Check sheet for the modelled part. Datum: model origin and axes. Units: mm. A direction names the side the tool comes from. Give positions to 0.01 mm unless a question says otherwise; leave off trailing zeros. Write each loop counter-clockwise with the first axis right and the second up, starting at its lowest first coordinate (ties: lowest second). Pieces come first, ordered by that corner, then holes. Notation, with made-up numbers: (-28, 27) -> (18, 27) arc R9 ccw to (18, 38) -> close; hole circle Ø11 at (-29, -31.5). An arc over 180 degrees is marked (long way). Answer as a JSON object with one key per item and string values.
from build123d import *

# Parameters (mm, degrees)
BOSS_EXTRUDE2_DEPTH = 3


with BuildPart() as part:
    # Sketch1 → Boss-Extrude2 (new body)
    with BuildSketch(Plane(origin=(0, 0, 0), x_dir=(1, 0, 0), z_dir=(0, 1, 0))):
        with BuildLine():
            Line((0, 0), (-3.8, 0))
            ThreePointArc((-3.8, 0), (-5.3, 1.5), (-3.8, 3))
            Line((-3.8, 3), (15.47, 3))
            Line((15.47, 3), (15.47, 4.149016738))
            ThreePointArc((15.47, 4.149016738), (14.185724127, 7.49466977), (10.992642316, 9.121626215))
            Line((10.992642316, 9.121626215), (5.783295319, 9.669150648))
            ThreePointArc((5.783295319, 9.669150648), (4.874143319, 10), (4.226657422, 10.718874584))
            ThreePointArc((4.226657422, 10.718874584), (-1.078837134, 13.36), (-5.3, 9.2))
            Line((-5.3, 9.2), (-8.03, 9.2))
            ThreePointArc((-8.03, 9.2), (-15.73, 1.5), (-8.03, -6.2))
            Line((-8.03, -6.2), (-1.5, -6.2))
            ThreePointArc((-1.5, -6.2), (-0.439339828, -5.760660172), (0, -4.7))
            Line((0, -4.7), (0, 0))
        make_face()
    extrude(amount=BOSS_EXTRUDE2_DEPTH)


solid = part.part
1. Sectioned sample at B-B, the plane z = -1.5. Enter the section's corners in (x, y), plus the area to 3 significant figures.
Determined:
{"outline": "(-15.73, 0) -> (-5.3, 0) -> (-5.3, 3) -> (-15.73, 3) -> close", "area": "31.3 mm^2"}
2. Scan lines: L1, parallel to Z at x = -2.5, y = 2.1; L2, parallel to Z at x = 5, y = 2.2; L3, parallel to X at y = 1.15, z = -3.25. Record each from-to range of solid material in increasing order. Write a range as [from, to].
Determined:
{"L1": "[-12.91, -3], [0, 6.2]", "L2": "[-9.92, -3]", "L3": "[-15.53, 15.47]"}
3. Access from +Z, -Z, +X, -X, +Y, -Y to the whole of each face (thin tool, end or side, straight path). Record for faces 1 (the face through (6, 1, -3)), 2 (the face through (-4, 3, -4)), 3 (the face through (4.89, 1.48, -9.99)), 4 (the face through (0, 1, 2)), 5 (the face through (-7, 1, -9.2)).
Determined:
{"face 1": "+X, +Y, -Y", "face 2": "+Z, -Z, +X, -X, +Y", "face 3": "-Z, +X, +Y, -Y", "face 4": "+Z, +X, +Y, -Y", "face 5": "-Z, -X, +Y, -Y"}
4. Mould release check, pull along Z, two halves, no side actions. Record for faces 6 (the face through (-5.3, 1.5, -1.5)), 7 (the face through (-15.73, 1.48, -1.67)), 8 (the face through (-0.45, 1.48, 5.77)), 9 (the face through (-2, 1, 0)): released by +Z, released by -Z, zero draft, split by the parting line, or undercut.
Determined:
{"face 6": "undercut", "face 7": "split by the parting line", "face 8": "released by +Z", "face 9": "undercut"}
5. Go/stop test with flat-tipped pins: P1, Ø1.4, axis at x = -6.5, y = 1, coming from the -Z side; P2, Ø1.5, axis at x = -2.5, y = 2, coming from the -Z side. Record where each tip stops, or that it passes through.
Determined:
{"P1": "z = -9.2", "P2": "z = -13.21"}
6. Sectioned sample at A-A, the plane y = 0.3. Enter the section's corners in (x, z), plus the area to 3 significant figures.
Determined:
{"outline": "(-8.03, -9.2) -> (-5.3, -9.2) arc R5.1 ccw to (4.23, -10.72) arc R2 cw to (5.78, -9.67) -> (10.99, -9.12) arc R5 ccw to (15.47, -4.15) -> (15.47, -3) -> (-3.8, -3) arc R1.5 cw to (-3.8, 0) -> (0, 0) -> (0, 4.7) arc R1.5 ccw to (-1.5, 6.2) -> (-8.03, 6.2) arc R7.7 ccw to start", "area": "325 mm^2"}
7. Sectioned sample at C-C, the plane x = 3.5. Enter the section's corners in (y, z).
Determined:
{"outline": "(0, -11.75) -> (3, -11.75) -> (3, -3) -> (0, -3) -> close"}
